Answer from the drawing. Dimensions are ordinates in mm from the lowest x, y and z of the part. Coordinates: 2 decimals unless noted, no trailing zeros. Order: outer loops, then holes, each group sorted by start corner. A loop starts at its lowest first (then second) coordinate and runs counter-clockwise, first axis right, second up. Notation, with made-up numbers: M 31.25,5.5 L 54.25,5.5 A19 cw 54.25,34.5 Z; hole C 56,-25.75 d7. An arc over 180 degrees is marked long. One line per question, with ' | ' between items. Start each with the question number.
1) Find section A-A, the plane z = 6.35. Write down the section's boundary in (x, y) (1 decimal).
2) Find section B-B, the plane x = 12.7. Write down the section's boundary in (y, z).
3) Given P1, Ø3, axis at x = 22.225, z = 15.875, coming from the +Y side; P2, Ø2, axis at x = 8, z = 7.5, coming from the -Y side, each flat-ended and moving along its own axis, determine where each tip first touches the part or whether it passes through.
4) Find section D-D, the plane y = 0.4. Count the separate pieces of the cut face and the enclosed holes in it, plus the area to 3 significant figures.
5) Consider probe 1 along Z at (x, y) = (12.5, 0.2); probe 2 along Z at (x, y) = (4, 0.4) (1 decimal); probe 3 along Z at (x, y) = (3.5, 0.6) (1 decimal). Determine where each line is inside the solid, lowest interval first.
6) Find section C-C, the plane z = 25.4. Write down the section's boundary in (x, y).
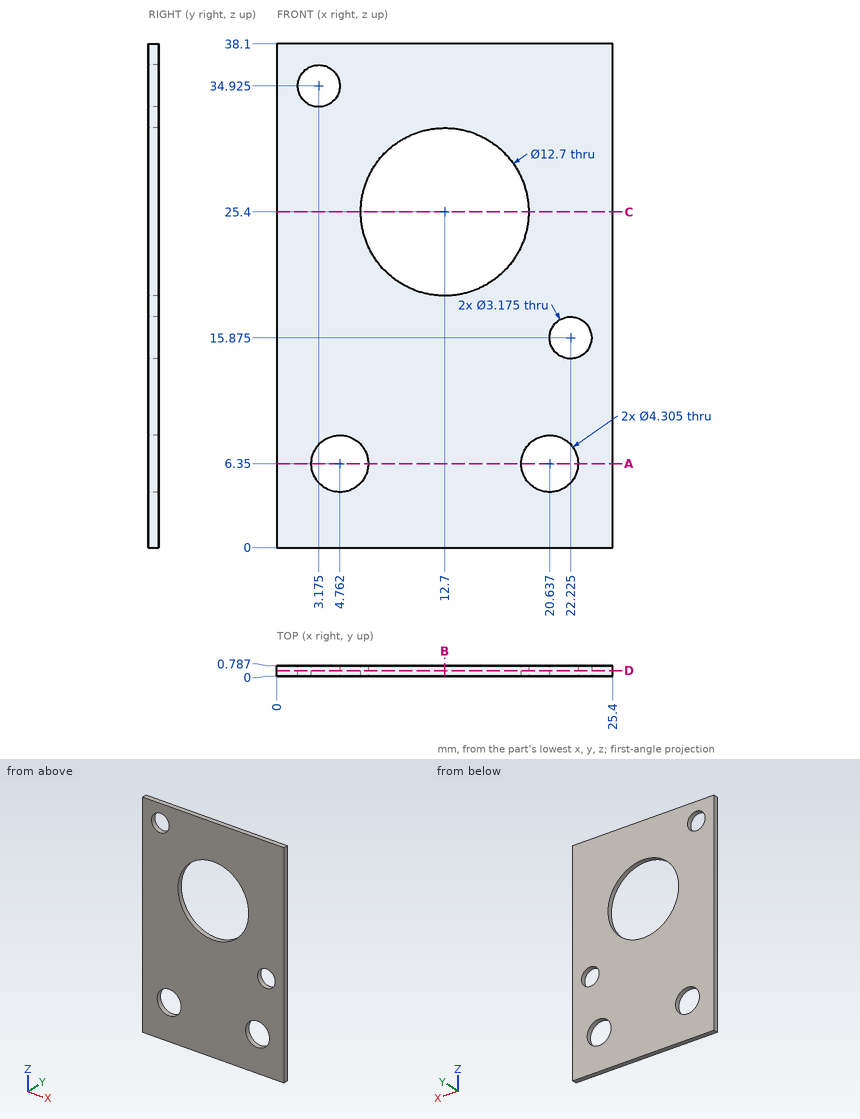
Report:
1) outline: M 0,0 L 2.6,0 L 2.6,0.8 L 0,0.8 Z; M 6.9,0 L 18.5,0 L 18.5,0.8 L 6.9,0.8 Z; M 22.8,0 L 25.4,0 L 25.4,0.8 L 22.8,0.8 Z
2) outline: M 0,0 L 0.79,0 L 0.79,19.05 L 0,19.05 Z; M 0,31.75 L 0.79,31.75 L 0.79,38.1 L 0,38.1 Z
3) P1: passes through | P2: stops at y = 0
4) separate pieces: 1 | enclosed holes: 5 | area: 796 mm^2
5) probe 1: z = 0 to 19.05, 31.75 to 38.1 | probe 2: z = 0 to 4.3, 8.4 to 33.6, 36.3 to 38.1 | probe 3: z = 0 to 4.6, 8.1 to 33.4, 36.5 to 38.1
6) outline: M 0,0 L 6.35,0 L 6.35,0.79 L 0,0.79 Z; M 19.05,0 L 25.4,0 L 25.4,0.79 L 19.05,0.79 Z
